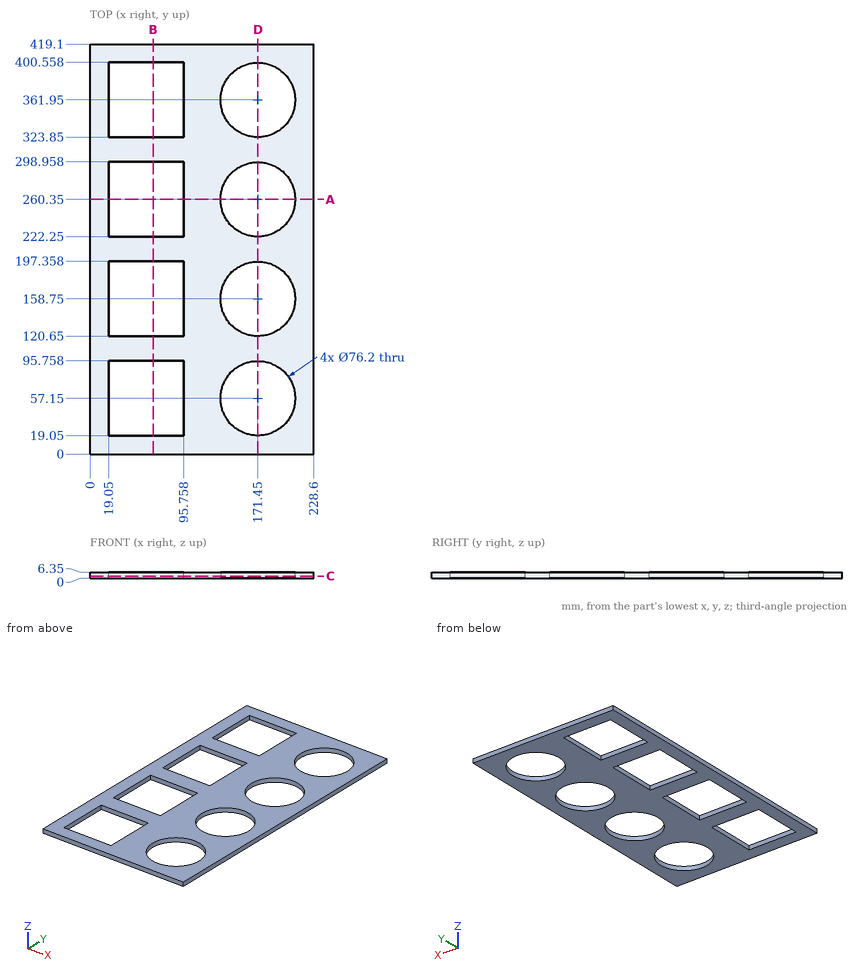
Source: three-view drawing plus pictorial views. Frame: mm from the lowest corner of the part. Coordinates: 2 decimals unless noted, no trailing zeros. Order: outer loops, then holes, each group sorted by start corner. A loop starts at its lowest first (then second) coordinate and runs counter-clockwise, first axis right, second up.
1) Section C-C (z = 2.5). Give the number of separate pieces and of enclosed holes in the cut face, then the cut area to 3 significant figures.
Result sheet:
separate pieces: 1
enclosed holes: 8
area: 54,000 mm2
2) Section B-B (x = 64.5). Return loops of the section in (y, z), then the cut area to 3 significant figures.
Result sheet:
outline: (0, 0) - (19.05, 0) - (19.05, 6.35) - (0, 6.35) - close; (95.76, 0) - (120.65, 0) - (120.65, 6.35) - (95.76, 6.35) - close; (197.36, 0) - (222.25, 0) - (222.25, 6.35) - (197.36, 6.35) - close; (298.96, 0) - (323.85, 0) - (323.85, 6.35) - (298.96, 6.35) - close; (400.56, 0) - (419.1, 0) - (419.1, 6.35) - (400.56, 6.35) - close
area: 713 mm2
3) Section D-D (x = 171.45). Return loops of the section in (y, z), then the cut area to 3 significant figures.
Result sheet:
outline: (0, 0) - (19.05, 0) - (19.05, 6.35) - (0, 6.35) - close; (95.25, 0) - (120.65, 0) - (120.65, 6.35) - (95.25, 6.35) - close; (196.85, 0) - (222.25, 0) - (222.25, 6.35) - (196.85, 6.35) - close; (298.45, 0) - (323.85, 0) - (323.85, 6.35) - (298.45, 6.35) - close; (400.05, 0) - (419.1, 0) - (419.1, 6.35) - (400.05, 6.35) - close
area: 726 mm2
4) Ray query, probe 1 along Y at (x, z) = (174, 0.5); probe 2 along X at (y, z) = (158.75, 5.25); probe 3 along Y at (x, z) = (79, 2). Return the intervals inside material, ascending.
Result sheet:
probe 1: y = 0 to 19.14, 95.16 to 120.74, 196.76 to 222.34, 298.36 to 323.94, 399.96 to 419.1
probe 2: x = 0 to 19.05, 95.76 to 133.35, 209.55 to 228.6
probe 3: y = 0 to 19.05, 95.76 to 120.65, 197.36 to 222.25, 298.96 to 323.85, 400.56 to 419.1
5) Section A-A (y = 260.35). Return loops of the section in (x, z), then the cut area to 3 significant figures.
Result sheet:
outline: (0, 0) - (19.05, 0) - (19.05, 6.35) - (0, 6.35) - close; (95.76, 0) - (133.35, 0) - (133.35, 6.35) - (95.76, 6.35) - close; (209.55, 0) - (228.6, 0) - (228.6, 6.35) - (209.55, 6.35) - close
area: 481 mm2
